The model under review builds one solid part; all positions refer to its coordinate system, in mm. A direction names the side the tool comes from. Coordinates: 2 decimals unless noted, no trailing zeros. Write each loop counter-clockwise with the first axis right and the second up, starting at its lowest first coordinate (ties: lowest second). Pieces come first, ordered by that corner, then holes. Notation, with made-up numbers: M 24.5,-19 L 67.5,-19 A13 cw 67.5,-2 Z; hole C 3.5,82.5 d10. An arc over 180 degrees is marked long. Answer as a JSON object with one key per item and string values.
Autodesk Inventor part; units mm, degrees
ref_plane "YZ Plane" through (0, 0, 0) normal (1, 0, 0) x (0, 1, 0)
ref_plane "XZ Plane" through (0, 0, 0) normal (0, 1, 0) x (-1, 0, 0)
ref_plane "XY Plane" through (0, 0, 0) normal (0, 0, 1) x (1, 0, 0)
sketch "Эскиз1" plane through (0, 0, 0) normal (0, 0, 1) x (1, 0, 0)
  line L0 (-19, 24) -> (19, 24)
  line L1 (19, 24) -> (19, -24)
  line L2 (19, -24) -> (-19, -24)
  line L3 (-19, -24) -> (-19, 24)
  line L4 (-19, 24) -> (19, -24) construction
  line L5 (19, 24) -> (-19, -24) construction
  line L6 (-101, 19) -> (101, 19)
  line L7 (101, 19) -> (101, -1)
  line L8 (101, -1) -> (-101, -1)
  line L9 (-101, -1) -> (-101, 19)
  point P0 (0, 0)
  point P1 (0, 0)
  point P2 (0, -1)
  point P3 (0, 0)
  dimension "d1" = 38
  dimension "d2" = 48
  dimension "d3" = 202
  dimension "d4" = 40
  dimension "d75" = 25
extrude "Выдавливание1" add sketch "Эскиз1" along normal mid plane 80 contours L0 L1 L6 L3 | L6 L1 L8 L3 | L8 L1 L2 L3
revolve "Вращение1" add sketch "Эскиз1" angle 360 about axis through (101, -1, 0) along (-1, 0, 0) contours L6 L1 L8 L3 | L3 L8 L9 L6 | L6 L7 L8 L1
hole "Отверстие1" at (-101, -1, 0) direction (1, 0, 0) diameter 27 end through all
hole "Отверстие2" at (0, -1, -40) direction (0, 0, 1) diameter 24 end up to surface
hole "Отверстие3" at (0, -1, 40) direction (0, 0, -1) diameter 8.376 end up to surface
hole "Отверстие4" at (0, 24, 0) direction (0, -1, 0) diameter 13.835 end up to surface
sketch "Эскиз2" plane through (0, 0, -40) normal (0, 0, -1) x (-1, 0, 0)
  circle A0 centre (0, -1) radius 12
  point P0 (12, 15)
  point P1 (-12, -17)
  point P2 (-12, 15)
  dimension "d71" = 12
  dimension "d73" = 16
  dimension "d76" = 32
  dimension "d77" = 12
hole "Отверстие5" at (-12, 15, -40) at (12, -17, -40) direction (0, 0, 1) diameter 4.917 depth 14 tip angle 118
hole "Отверстие6" at (12, 15, -40) direction (0, 0, 1) diameter 8 depth 22 tip angle 118
chamfer "Фаска1" distance 1 angle 45 2 edges at (-12, 12.5415, -40) (12, -19.4585, -40)
chamfer "Фаска2" distance 1.6 angle 45 1 edges at (12, 11, -40)
properties part number "Колонка"
(1) Add section D-D on z = -30.5. Give the boundary of the cut face in (x, y), and give its area (3 significant figures).
Results list:
{"outline": "M -19,-24 L 19,-24 L 19,24 L -19,24 Z; hole C -12,15 d4.92; hole C 0,-1 d24; hole C 12,15 d8; hole C 12,-17 d4.92", "area": "1,280 mm²"}
(2) For pin 1 Ø6 at (y, z) = (18.5, 15) entering from -X; pin 2 Ø5.5 at (x, y) = (-12, 15) entering from -Z; pin 3 Ø21.5 at (x, y) = (0, -1) entering from -Z; pin 4 Ø16 at (y, z) = (-1, 0) entering from +X, all flat-tipped, find the tip position at first contact; note any pin that passes through.
Results list:
{"pin 1": "x = -19", "pin 2": "z = -39.29", "pin 3": "z = 8.17", "pin 4": "through"}
(3) Add section A-A on y = -1. Give the boundary of the cut face in (x, z), and give its area (3 significant figures).
Results list:
{"outline": "M -101,-20 L -19,-20 L -19,-40 L -12,-40 L -12,-13.5 L -101,-13.5 Z; M -101,13.5 L -4.19,13.5 L -4.19,40 L -19,40 L -19,20 L -101,20 Z; M 4.19,13.5 L 101,13.5 L 101,20 L 19,20 L 19,40 L 4.19,40 Z; M 12,-40 L 19,-40 L 19,-20 L 101,-20 L 101,-13.5 L 12,-13.5 Z", "area": "3,290 mm²"}
(4) For faces 1 (the face through (-13.662, 13.188, -32.409)), 2 (the face through (60.57, -20.98, 0.88)), 3 (the face through (-59.43, -20.98, 0.88)), list the 3-axis set-ups (+Z, -Z, +X, -X, +Y, -Y) from which the entire face can be reached by the end or side of a thin tool; tool diameter is ignored.
Results list:
{"face 1": "-Z", "face 2": "+X", "face 3": "-X"}
(5) Add section C-C on x = 0. Give the boundary of the cut face in (y, z), and give its area (3 significant figures).
Results list:
{"outline": "M -24,-40 L -13,-40 L -13,-6.18 A13.5 cw -5.19,12.83 L -5.19,40 L -24,40 Z; M 3.19,12.83 A13.5 cw 10.59,6.92 L 24,6.92 L 24,40 L 3.19,40 Z; M 11,-40 L 24,-40 L 24,-6.92 L 11,-6.92 Z", "area": "2,190 mm²"}
(6) Add section B-B on z = 0. Give the boundary of the cut face in (x, y).
Results list:
{"outline": "M -101,-21 L -19,-21 L -19,-24 L 19,-24 L 19,-21 L 101,-21 L 101,-14.5 L -101,-14.5 Z; M -101,12.5 L -6.92,12.5 L -6.92,24 L -19,24 L -19,19 L -101,19 Z; M 6.92,12.5 L 101,12.5 L 101,19 L 19,19 L 19,24 L 6.92,24 Z"}
(7) Wall thickness on line 1 along X through (y, z) = (15, -35); line 2 along Y through (x, z) = (0, 34.5); line 3 along Y through (x, z) = (0, -32): over which ranges is each line inside the solid? List them lowest first. Write a range as from..to.
Results list:
{"line 1": "-19..-14.46, -9.54..8, 16..19", "line 2": "-24..-5.19, 3.19..24", "line 3": "-24..-13, 11..24"}
(8) Draft analysis for pull direction X (two halves, no side actions). For faces 4 (the face through (-19, 10, -18)), 5 (the face through (11.62, -16.8, -24.78)), 6 (the face through (-13, 0, -40)), state which applies: released by +X, released by -X, zero draft, split by the parting line, or undercut.
Results list:
{"face 4": "released by -X", "face 5": "undercut", "face 6": "zero draft"}
